Could you check a few things on this model? Use its own coordinates, in mm. A direction names the side the tool comes from. Give positions to 0.01 mm unless a question says otherwise; leave off trailing zeros. Loops run counter-clockwise (first coordinate to the right, second up) from the corner with the lowest first, then second, coordinate; pieces in that order, holes last. Notation, with made-up numbers: (76.25, -6.5) - (85.25, -6.5) arc R16 ccw to (85.25, 9.5) - close; hole circle Ø10 at (45, 65.5). An arc over 180 degrees is marked (long way). Answer in a Markdown table with one row per item. Add a question column.
```python
from build123d import *

# Parameters (mm, degrees)
RESSALTO_EXTRUS_O1_DEPTH = 10
ESBO_O2_R                = 2.5
CORTE_EXTRUS_O1_DEPTH    = 10
FILETE1_R                = 5
CORTE_EXTRUS_O4_DEPTH    = 10
CORTE_EXTRUS_O5_DEPTH    = 10
ESBO_O7_R                = 3.175
RESSALTO_EXTRUS_O2_DEPTH = 0.1


with BuildPart() as part:
    # Esboço1 → Ressalto-extrusão1 (new body)
    with BuildSketch(Plane.XY):
        Polygon((-10, -7.5), (20, 15), (-10, 15), (-10, 4.8), (-20, 4.8), (-20, -4.8), (-10, -4.8), align=None)
        Polygon((20, -15), (20, 15), (-10, -7.5), (-10, -15), align=None)
    extrude(amount=RESSALTO_EXTRUS_O1_DEPTH)

    # Esboço2 → Corte-extrusão1 (cut)
    with BuildSketch(Plane.XZ.offset(4.8)):
        with Locations(Location((-15, 5, 0), (0, 0, 270))):
            Circle(ESBO_O2_R)
    extrude(amount=-CORTE_EXTRUS_O1_DEPTH, mode=Mode.SUBTRACT)

    # Filete1
    filete1_edges = [part.edges().sort_by_distance(p)[0] for p in [
        (-20, 0, 0),
        (-20, 0, 10),
    ]]
    fillet(filete1_edges, radius=FILETE1_R - 0.0001)  # a hair under: the kernel refuses the full size

    # Esboço5 → Corte-extrusão4 (cut)
    with BuildSketch(Plane.XZ.offset(15)):
        with BuildLine():
            Line((-10, 10), (-10, 0))
            ThreePointArc((-10, 0), (-9.341737512, 5), (-10, 10))
        make_face()
    extrude(amount=-CORTE_EXTRUS_O4_DEPTH, mode=Mode.SUBTRACT)

    # Esboço6 → Corte-extrusão5 (cut)
    with BuildSketch(Plane(origin=(0, 15, 0), x_dir=(1, 0, 0), z_dir=(0, 1, 0))):
        with BuildLine():
            Line((-10, -9.950546275), (-10, 0))
            ThreePointArc((-10, 0), (-9.344992865, -4.975273137), (-10, -9.950546275))
        make_face()
    extrude(amount=-CORTE_EXTRUS_O5_DEPTH, mode=Mode.SUBTRACT)

    # Esboço7 → Ressalto-extrusão2 (add)
    with BuildSketch(Plane.XY.offset(10)):
        with Locations((5, 0)):
            Circle(ESBO_O7_R)
    extrude(amount=RESSALTO_EXTRUS_O2_DEPTH)


solid = part.part
```
(1) We'd pull the mould along Z, two halves only. Please class faces 1 (the flat face through (-12, -4.8, 5)), 2 (the flat face through (2, 0, 0)), 3 (the cylindrical face through (-9.34, -10.07, 4.93)), 4 (the cylindrical face through (-15.96, -0.07, 2.69)): pulls with the +Z half, pulls with the -Z half, needs draft (parallel to the pull), parting line crosses it, or undercut.
(2) On a 3-axis mill with a long thin cutter (end or side, diameter ignored), from which of +Z, -Z, +X, -X, +Y, -Y can I reach the whole of each face in a straight line? I mean faces 5 (the flat face through (5, 15, 5)), 6 (the flat face through (-13, 4.8, 3)), 7 (the cylindrical face through (-9.345, 10.07, 4.905)). Say none if no direction works.
(3) I want a section at D-D on z = 6.25. Please give me the cut outline in (x, y), then the cut area to 3 significant figures.
(4) I want a section at C-C on y = 13. Please give me the cut outline in (x, z), then the cut area to 3 significant figures.
(5) Please list where these lines run through material, in increasing order: line 1 (X direction, y = 1, z = 5); line 2 (Z direction, x = 16.5, y = 11.5); line 3 (Y direction, x = -18, z = 2).
(6) For pin 1 Ø0.7 at (x, z) = (-9.5, 6.5) entering from -Y; pin 2 Ø6 at (y, z) = (10, 5) entering from -X; pin 3 Ø3 at (x, z) = (-15, 5) entering from -Y; pin 4 Ø3 at (y, z) = (10, 5.5) entering from -X, each with a flat end and sliding along its axis, tell me the tip position at first contact or that it passes through.
(7) I want a section at B-B on z = 3.5. Please give me the cut outline in (x, y).
Reported:
| question | item | result |
|---|---|---|
| 1 | face 1 | needs draft |
| 1 | face 2 | pulls with the -Z half |
| 1 | face 3 | undercut |
| 1 | face 4 | undercut |
| 2 | face 5 | +Z, -Z, +X, -X, +Y |
| 2 | face 6 | +Z, -Z, -X, +Y |
| 2 | face 7 | -X, +Y |
| 3 | outline | (-19.84, -4.8) - (-17.17, -4.8) - (-17.17, 4.8) - (-19.84, 4.8) - close; (-12.83, -4.8) - (-10, -4.8) - (-10, -5) - (-9.38, -5) - (-9.38, -15) - (20, -15) - (20, 15) - (-9.39, 15) - (-9.39, 5) - (-10, 5) - (-10, 4.8) - (-12.83, 4.8) - close |
| 3 | area | 941 mm² |
| 4 | outline | (-10, 0) - (20, 0) - (20, 10) - (-10, 10) - (-10, 9.95) arc R19.22 cw to start |
| 4 | area | 296 mm² |
| 5 | line 1 | -20 to -17.5, -12.5 to 20 |
| 5 | line 2 | 0 to 10 |
| 5 | line 3 | -4.8 to 4.8 |
| 6 | pin 1 | y = -15 |
| 6 | pin 2 | x = -9.58 |
| 6 | pin 3 | through |
| 6 | pin 4 | x = -9.45 |
| 7 | outline | (-19.77, -4.8) - (-17, -4.8) - (-17, 4.8) - (-19.77, 4.8) - close; (-13, -4.8) - (-10, -4.8) - (-10, -5) - (-9.4, -5) - (-9.4, -15) - (20, -15) - (20, 15) - (-9.4, 15) - (-9.4, 5) - (-10, 5) - (-10, 4.8) - (-13, 4.8) - close |
